The model under review builds one solid part; all positions refer to its coordinate system, in mm. A direction names the side the tool comes from. Coordinates: 2 decimals unless noted, no trailing zeros. Order: outer loops, then holes, each group sorted by start corner. A loop starts at its lowest first (then second) coordinate and runs counter-clockwise, first axis right, second up. Notation, with made-up numbers: (19.25, -5.5) -> (55.25, -5.5) arc R25 cw to (55.25, 10.5) -> close; hole circle Ø1 at (33, 4.5). An arc over 180 degrees is marked (long way). Use one line per item in the form item = value.
from build123d import *

# Parameters (mm, degrees)
SKETCH2_R           = 76
BOSS_EXTRUDE1_DEPTH = 17.78
CUT_EXTRUDE3_DEPTH  = 13.97
CUT_EXTRUDE4_DEPTH  = 14.97
CUT_EXTRUDE5_DEPTH  = 1.27
SKETCH10_W          = 10.16
SKETCH10_H          = 41.91
SKETCH10_W_2        = 41.91
SKETCH10_H_2        = 10.16
CUT_EXTRUDE6_DEPTH  = 1.016
SKETCH11_W          = 44.45
SKETCH11_H          = 44.45
BOSS_EXTRUDE2_DEPTH = 1.27
SKETCH14_R          = 3.175
BOSS_EXTRUDE4_DEPTH = 5.08
SKETCH15_R          = 73.66
BOSS_EXTRUDE5_DEPTH = 2.54


with BuildPart() as part:
    # Sketch2 → Boss-Extrude1 (new body)
    with BuildSketch(Plane(origin=(0, 0, 0), x_dir=(1, 0, 0), z_dir=(0, 1, 0))):
        Circle(SKETCH2_R)
    extrude(amount=BOSS_EXTRUDE1_DEPTH)

    # Sketch6 → Cut-Extrude3 (cut)
    with BuildSketch(Plane(origin=(0, 17.78, 0), x_dir=(1, 0, 0), z_dir=(0, 1, 0))):
        with BuildLine():
            Line((-76, 35.56), (76, 35.56))
            ThreePointArc((76, 35.56), (111.56, 0), (76, -35.56))
            Line((76, -35.56), (-76, -35.56))
            ThreePointArc((-76, -35.56), (-111.56, 0), (-76, 35.56))
        make_face()
    extrude(amount=-CUT_EXTRUDE3_DEPTH, mode=Mode.SUBTRACT)

    # Sketch8 → Cut-Extrude4 (cut, through all)
    with BuildSketch(Plane(origin=(0, 3.81, 0), x_dir=(1, 0, 0), z_dir=(0, 1, 0))):
        with BuildLine():
            Line((35.56, 76), (35.56, -76))
            ThreePointArc((35.56, -76), (0, -111.56), (-35.56, -76))
            Line((-35.56, -76), (-35.56, 76))
            ThreePointArc((-35.56, 76), (0, 111.56), (35.56, 76))
        make_face()
    extrude(amount=CUT_EXTRUDE4_DEPTH, mode=Mode.SUBTRACT)

    # Sketch9 → Cut-Extrude5 (cut)
    with BuildSketch(Plane(origin=(0, 3.81, 0), x_dir=(1, 0, 0), z_dir=(0, 1, 0))):
        with BuildLine():
            Line((25.4, 76), (25.4, 25.4))
            Line((25.4, 25.4), (76, 25.4))
            ThreePointArc((76, 25.4), (101.4, 0), (76, -25.4))
            Line((76, -25.4), (25.4, -25.4))
            Line((25.4, -25.4), (25.4, -76))
            ThreePointArc((25.4, -76), (0, -101.4), (-25.4, -76))
            Line((-25.4, -76), (-25.4, -25.4))
            Line((-25.4, -25.4), (-76, -25.4))
            ThreePointArc((-76, -25.4), (-101.4, 0), (-76, 25.4))
            Line((-76, 25.4), (-25.4, 25.4))
            Line((-25.4, 25.4), (-25.4, 76))
            ThreePointArc((-25.4, 76), (0, 101.4), (25.4, 76))
        make_face()
    extrude(amount=-CUT_EXTRUDE5_DEPTH, mode=Mode.SUBTRACT)

    # Sketch10 → Cut-Extrude6 (cut)
    with BuildSketch(Plane(origin=(0, 2.54, 0), x_dir=(1, 0, 0), z_dir=(0, 1, 0))):
        with Locations((-14.037724316, 46.60290417)):
            Rectangle(SKETCH10_W, SKETCH10_H)
        with Locations((14.037724316, 46.60290417)):
            Rectangle(SKETCH10_W, SKETCH10_H)
        with Locations((14.037724316, -46.60290417)):
            Rectangle(SKETCH10_W, SKETCH10_H)
        with Locations((-14.037724316, -46.60290417)):
            Rectangle(SKETCH10_W, SKETCH10_H)
        with Locations((-48.79885899, 13.97)):
            Rectangle(SKETCH10_W_2, SKETCH10_H_2)
        with Locations((-48.79885899, -13.97)):
            Rectangle(SKETCH10_W_2, SKETCH10_H_2)
        with Locations((48.79885899, -13.97)):
            Rectangle(SKETCH10_W_2, SKETCH10_H_2)
        with Locations((48.79885899, 13.97)):
            Rectangle(SKETCH10_W_2, SKETCH10_H_2)
    extrude(amount=-CUT_EXTRUDE6_DEPTH, mode=Mode.SUBTRACT)

    # Sketch11 → Boss-Extrude2 (add)
    with BuildSketch(Plane(origin=(0, 2.54, 0), x_dir=(1, 0, 0), z_dir=(0, 1, 0))):
        Rectangle(SKETCH11_W, SKETCH11_H)
    extrude(amount=BOSS_EXTRUDE2_DEPTH)

    # Sketch14 → Boss-Extrude4 (add)
    with BuildSketch(Plane(origin=(0, 3.81, 0), x_dir=(1, 0, 0), z_dir=(0, 1, 0))):
        Circle(SKETCH14_R)
    extrude(amount=BOSS_EXTRUDE4_DEPTH)

    # Sketch15 → Boss-Extrude5 (add)
    with BuildSketch(Plane.XZ):
        Circle(SKETCH15_R)
    extrude(amount=BOSS_EXTRUDE5_DEPTH)


solid = part.part
Item 1: To check wall thickness, follow L1, parallel to X at y = 2.5, z = -14; L2, parallel to Y at x = 17, z = -60; L3, parallel to X at y = 2.75, z = -44.5. State the ranges of each line that lie inside material, in increasing order. Write a range as from..to.
Results found:
L1 = -74.7..-69.75, -27.84..27.84, 69.75..74.7
L2 = -2.54..1.52
L3 = -61.61..-25.4, 25.4..61.61
Item 2: Draft analysis for pull direction X (two halves, no side actions). For faces 1 (the face through (49, 1.524, -14)), 2 (the face through (52, 11, 35.56)), 3 (the face through (-58.454, -1.252, -44.821)), state which applies: released by +X, released by -X, zero draft, split by the parting line, or undercut.
Results found:
face_1 = undercut
face_2 = zero draft
face_3 = split by the parting line
Item 3: We need section B-B (x = 0). Write out the cut boundary in (y, z) (3 decimals), plus the area to 3 significant figures.
Results found:
outline = (-2.54, -73.66) -> (0, -73.66) -> (0, -76) -> (2.54, -76) -> (2.54, -22.225) -> (3.81, -22.225) -> (3.81, -3.175) -> (8.89, -3.175) -> (8.89, 3.175) -> (3.81, 3.175) -> (3.81, 22.225) -> (2.54, 22.225) -> (2.54, 76) -> (0, 76) -> (0, 73.66) -> (-2.54, 73.66) -> close
area = 849 mm²
Item 4: Clearance check with flat-ended pins moving along their axes: pin 1 (1 mm diameter, centred on x = 42, y = 3, fed in from +Z); pin 2 (0.8 mm diameter, centred on y = 2, z = -11.5, fed in from -X); pin 3 (0.5 mm diameter, centred on x = 53, y = 2, fed in from -Z). State where each tip first meets the part, or that it passes through.
Results found:
pin_1 = 63.67
pin_2 = -75.19
pin_3 = -54.71
Item 5: Tool access review of faces 4 (the face through (-35.56, 11, 52)), 5 (the face through (51, 11, -35.56)), 6 (the face through (48, 17.78, -48)), 7 (the face through (-49, 1.524, 14)): name each direction out of +Z, -Z, +X, -X, +Y, -Y from which nothing blocks a thin tool from reaching the whole face with its end or side.
Results found:
face_4 = +Z, -Z, +Y
face_5 = +X, -X, +Y
face_6 = +Z, -Z, +X, -X, +Y
face_7 = +Y
Item 6: We need section C-C (y = 7). Write out the cut boundary in (x, z) (3 decimals).
Results found:
outline = (-67.168, -35.56) arc R76 ccw to (-35.56, -67.168) -> (-35.56, -35.56) -> close; (-67.168, 35.56) -> (-35.56, 35.56) -> (-35.56, 67.168) arc R76 ccw to start; circle Ø6.35 at (0, 0); (35.56, -67.168) arc R76 ccw to (67.168, -35.56) -> (35.56, -35.56) -> close; (35.56, 35.56) -> (67.168, 35.56) arc R76 ccw to (35.56, 67.168) -> close
Item 7: We need section A-A (y = 15.25). Write out the cut boundary in (x, z).
Results found:
outline = (-67.17, -35.56) arc R76 ccw to (-35.56, -67.17) -> (-35.56, -35.56) -> close; (-67.17, 35.56) -> (-35.56, 35.56) -> (-35.56, 67.17) arc R76 ccw to start; (35.56, -67.17) arc R76 ccw to (67.17, -35.56) -> (35.56, -35.56) -> close; (35.56, 35.56) -> (67.17, 35.56) arc R76 ccw to (35.56, 67.17) -> close
Item 8: We need section D-D (z = 0). Write out the cut boundary in (x, y) (3 decimals), plus the area to 3 significant figures.
Results found:
outline = (-76, 0) -> (-73.66, 0) -> (-73.66, -2.54) -> (73.66, -2.54) -> (73.66, 0) -> (76, 0) -> (76, 2.54) -> (22.225, 2.54) -> (22.225, 3.81) -> (3.175, 3.81) -> (3.175, 8.89) -> (-3.175, 8.89) -> (-3.175, 3.81) -> (-22.225, 3.81) -> (-22.225, 2.54) -> (-76, 2.54) -> close
area = 849 mm²
